```python
from build123d import *

# Parameters (mm, degrees)
F0_W     = 71.5159550309
F0_H     = 51.0343238711
F1_DEPTH = 25
F2_R     = 25
F3_DEPTH = 88
F4_R     = 50.4354263915
F5_DEPTH = 25


with BuildPart() as f1:
    # F0 (on Front) → F1 (new body)
    with BuildSketch(Plane.XZ):
        with Locations((35.7579775155, 25.5171619356)):
            Rectangle(F0_W, F0_H)
    extrude(amount=F1_DEPTH)

    # F2 (on Right) → F3 (join)
    with BuildSketch(Plane.YZ):
        with Locations((1.7605778567, 19.9215863818)):
            Circle(F2_R)
    extrude(amount=F3_DEPTH)

    # F4 (on Front) → F5 (join)
    with BuildSketch(Plane.XZ):
        with Locations((67.9112821817, 44.1088192165)):
            Circle(F4_R)
    extrude(amount=F5_DEPTH)


solid = f1.part
```
Work out the finished part from the listing and answer in its coordinate system (mm). A direction names the side the tool comes from. Give positions to 0.01 mm unless a question says otherwise; leave off trailing zeros. Order: outer loops, then holes, each group sorted by start corner. A loop starts at its lowest first (then second) coordinate and runs counter-clockwise, first axis right, second up. Notation, with made-up numbers: (21, 60.25) -> (66, 60.25) arc R11 cw to (66, 66.25) -> close; hole circle Ø5 at (14.25, 50.25). An arc over 180 degrees is marked (long way). Answer as CSV lines item,"result". Start each with the question number.
(1) Consider line 1 along Z through (x, y) = (87.5, 2.5); line 2 along Y through (x, z) = (69, 83); line 3 along Z through (x, y) = (16.5, -15). Determine where each line is inside the solid, lowest interval first.
(2) Section B-B, the plane x = 59.5 is taken. Write down the section's boundary in (y, z).
(3) Section D-D, the plane z = 80 is taken. Write down the section's boundary in (x, y), plus the area to 3 significant figures.
(4) Each of these flat-tipped pins is pushed along its axis until it touches: pin 1 Ø3 at (y, z) = (20, 33.5) entering from +X; pin 2 Ø8 at (y, z) = (-13.5, 55.5) entering from -X; pin 3 Ø3 at (x, z) = (51, 6) entering from +Y; pin 4 Ø1.5 at (y, z) = (2, 65) entering from +X. Where does it stop, or does it pass through?
(5) Section A-A, the plane y = -4 is taken. Write down the section's boundary in (x, z).
(6) Section C-C, the plane z = 15 is taken. Write down the section's boundary in (x, y), plus the area to 3 significant figures.
(7) Which of the six approach directions +Z, -Z, +X, -X, +Y, -Y give full straight-line access (tool end or side, diameter ignored) to faces 1 (the flat face through (9, -12, 51.034)), 2 (the flat face through (58, -25, 45)), 3 (the flat face through (0, 1, 23)), 4 (the flat face through (21, -19, 0)), 5 (the cylindrical face through (113.801, -12.325, 65.034))?
Entries:
1,line 1,"-5.07 to 44.91"
1,line 2,"-25 to 0"
1,line 3,"0 to 51.03"
2,outline,"(-25, -5.62) -> (0, -5.62) -> (0, -5.02) arc R25 ccw (long way) to (0, 44.86) -> (0, 93.84) -> (-25, 93.84) -> close"
3,outline,"(32.48, -25) -> (103.35, -25) -> (103.35, 0) -> (32.48, 0) -> close"
3,area,"1,770 mm²"
4,pin 1,"x = 88"
4,pin 2,"x = 18.02"
4,pin 3,"y = 23.46"
4,pin 4,"through"
5,outline,"(0, -4.41) -> (54.12, -4.41) arc R50.44 ccw to (81.7, -4.41) -> (88, -4.41) -> (88, -2.15) arc R50.44 ccw (long way) to (17.95, 51.03) -> (0, 51.03) -> close"
6,outline,"(0, -25) -> (109.1, -25) -> (109.1, 0) -> (88, 0) -> (88, 26.27) -> (0, 26.27) -> close"
6,area,"5,040 mm²"
7,face 1,"+Z, -X, +Y, -Y"
7,face 2,"+Z, -Z, +X, -X, -Y"
7,face 3,"+Z, -Z, -X, +Y, -Y"
7,face 4,"-Z, -X, -Y"
7,face 5,"-Y"
